The model under review builds one solid part; all positions refer to its coordinate system, in mm. Face numbers are marked on the shaded views. A direction names the side the tool comes from. Give positions to 0.01 mm unless a question says otherwise; leave off trailing zeros. Loops run counter-clockwise (first coordinate to the right, second up) from the corner with the lowest first, then second, coordinate; pieces in that order, holes last. Notation, with made-up numbers: M 80.25,0.25 L 124.25,0.25 A21 ccw 124.25,22.25 Z; hole C -29.5,61.25 d3. An arc over 180 degrees is marked long. Put each result on its own line as item: value. Start each with the question number.
```python
from build123d import *

# Parameters (mm, degrees)
SKETCH_1_R               = 17.5
EXTRUDE_1_DEPTH          = 10
EXTRUDE_2_DEPTH          = 10
PATTERN_CIRCULAR_1_COUNT = 20
SKETCH_3_R               = 2.5
CUT_EXTRUDE_1_DEPTH      = 33.680269277


with BuildPart() as part:
    # Эскиз1 → Бобышка-Вытянуть1 (new body)
    with BuildSketch(Plane(origin=(0, 0, 0), x_dir=(1, 0, 0), z_dir=(0, 1, 0))):
        with Locations(Location((0, 0, 0), (0, 0, 270))):
            Circle(SKETCH_1_R)
    extrude(amount=EXTRUDE_1_DEPTH)

    # Эскиз2 → Бобышка-Вытянуть2 (add)
    with BuildSketch(Plane.XZ):
        with BuildLine():
            Line((-1.631691003, 17.423764934), (-1.752328912, 18.711978549))
            ThreePointArc((-1.752328912, 18.711978549), (-1.433460227, 20.418219236), (-0.694874519, 21.989023384))
            ThreePointArc((-0.694874519, 21.989023384), (0, 22), (0.694874519, 21.989023384))
            ThreePointArc((0.694874519, 21.989023384), (1.433460227, 20.418219236), (1.752328912, 18.711978549))
            Line((1.752328912, 18.711978549), (1.631691003, 17.423764934))
            ThreePointArc((1.631691003, 17.423764934), (0, 17.5), (-1.631691003, 17.423764934))
        make_face()
    extrude_2 = extrude(amount=-EXTRUDE_2_DEPTH)

    # Круговой массив1: Бобышка-Вытянуть2 ×20 about axis
    pattern_circular_1_axis = Axis((0, 0, 0), (0, 1, 0))
    for i in range(1, PATTERN_CIRCULAR_1_COUNT):
        add(extrude_2.rotate(pattern_circular_1_axis, i * 360 / PATTERN_CIRCULAR_1_COUNT))

    # Эскиз3 → Вырез-Вытянуть1 (cut, through all)
    with BuildSketch(Plane.XZ):
        with Locations(Location((0, 0, 0), (0, 0, 270))):
            Circle(SKETCH_3_R)
    extrude(amount=-CUT_EXTRUDE_1_DEPTH, mode=Mode.SUBTRACT)


solid = part.part
```
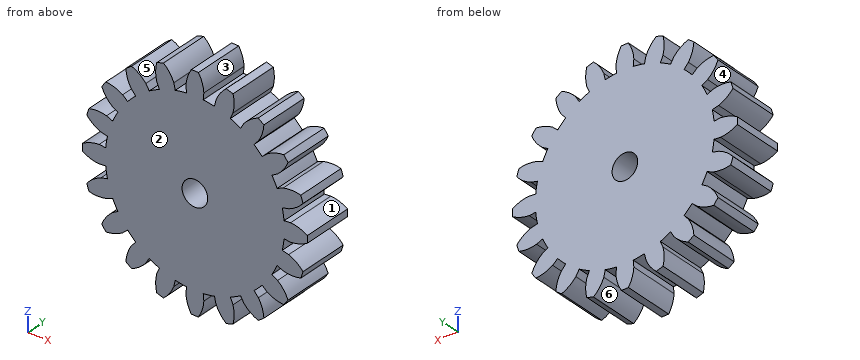
Item 1: Draft analysis for pull direction Z (two halves, no side actions). For the marked faces 1, 2 and 3, state which applies: +Z half, -Z half, draft (parallel to the pull), parting line (faces both ways), or undercut.
Item 2: Consider section C-C, the plane x = -11. Write out the cut boundary in (y, z).
Item 3: Consider section A-A, the plane x = 0. Write out the cut boundary in (y, z), plus the area to 3 significant figures.
Item 4: To check wall thickness, follow L1, parallel to X at y = 4, z = 0; L2, parallel to Z at x = -19.5, y = 8.25. State the ranges of each line that lie inside material, in increasing order. Write a range as [from, to].
Item 5: Consider section B-B, the plane z = 0. Write out the cut boundary in (x, y).
Item 6: Tool access review of the marked faces 4, 5 and 6: name each direction out of +Z, -Z, +X, -X, +Y, -Y from which nothing blocks a thin tool from reaching the whole face with its end or side.
Item 7: Clearance check with flat-ended pins moving along their axes: pin 1 Ø4 at (x, y) = (5, 3.5) entering from +Z; pin 2 Ø4 at (x, y) = (-13.5, 6.5) entering from +Z; pin 3 Ø8 at (x, z) = (16.5, 4.5) entering from -Y; pin 4 Ø3 at (x, z) = (0, 0) entering from -Y. State where each tip first meets the part, or that it passes through.
Report:
1. face 1: undercut
1. face 2: draft
1. face 3: +Z half
2. outline: M 0,-17.47 L 10,-17.47 L 10,17.47 L 0,17.47 Z
3. outline: M 0,-22 L 10,-22 L 10,-2.5 L 0,-2.5 Z; M 0,2.5 L 10,2.5 L 10,22 L 0,22 Z
3. area: 390 mm²
4. L1: [-22, -2.5], [2.5, 22]
4. L2: [-7.65, -4.7], [-1.66, 1.66], [4.7, 7.65]
5. outline: M -22,0 L -2.5,0 L -2.5,10 L -22,10 Z; M 2.5,0 L 22,0 L 22,10 L 2.5,10 Z
6. face 4: -X, +Y, -Y
6. face 5: +Z, +Y, -Y
6. face 6: -Z, +Y, -Y
7. pin 1: z = 21.13
7. pin 2: z = 18.2
7. pin 3: y = 0
7. pin 4: through
